Work out the finished part from the listing and answer in its coordinate system (mm). Coordinates: 2 decimals unless noted, no trailing zeros. Write each loop counter-clockwise with the first axis right and the second up, starting at its lowest first coordinate (ties: lowest second). Pieces come first, ordered by that corner, then holes. Notation, with made-up numbers: (88, 62.5) - (146, 62.5) arc R36 cw to (146, 100.5) - close; hole circle Ø7 at (-1.5, -17). An arc over 180 degrees is marked (long way). Use a Markdown table: item, result. Add a question column.
(1) The part is cut by section C-C, the plane z = -9. Give the vertices of the cut face in (x, y).
(2) The part is cut by section A-A, the plane y = 0.3. Give the vertices of the cut face in (x, z).
(3) For a pull along Y with two mould halves and no side action, classify faces 1 (the face through (-1, 1.016, -27)), 2 (the face through (-23.657, 0.751, 27.237)), 3 (the face through (-1, 0, -12)) as released by +Y, released by -Y, zero draft, split by the parting line, or undercut.
(4) Find the intervals of material crossed by line 1 (Y direction, x = -48, z = -41); line 2 (Z direction, x = 60, y = 0.5); line 3 (Z direction, x = -17, y = 0.2), in increasing order. Write a range as from..to.
(5) The part is cut by section D-D, the plane x = 32. Give the vertices of the cut face in (y, z).
(6) The part is cut by section B-B, the plane x = -10. Give the vertices of the cut face in (y, z), then the cut area to 3 significant figures.
(7) Given pin 1 Ø0.5 at (x, y) = (51, 0.5) entering from +Z; pin 2 Ø16.5 at (x, z) = (-21, -35.5) entering from +Y, each flat-ended and moving along its own axis, determine where each tip first touches the part or whether it passes through.
from build123d import *

# Parameters (mm, degrees)
F34_W     = 153.4406170249
F34_H     = 55.5722899735
F35_DEPTH = 0.762
F37_DEPTH = 1.27
F39_DEPTH = 0.254
F40_DEPTH = 0.254


# Not quite as in the source:
# - the program builds the solid bodies; features that only make, move or delete a surface that nothing else refers to are left out


with BuildPart() as f35:
    # F34 (on Front) → F35 (new body)
    with BuildSketch(Plane.XZ):
        with Locations((0.281136483, -27.7861449867)):
            Rectangle(F34_W, F34_H)
    extrude(amount=-F35_DEPTH)

    # F36 (on Front) → F37 (join)
    with BuildSketch(Plane.XZ):
        Polygon((41.6817590594, 0), (0, 55.2465841174), (-46.6600246727, 0), align=None)
    extrude(amount=-F37_DEPTH)

    # F38 (on face) → F39 (join)
    with BuildSketch(Plane(origin=(0, 1.27, 0), x_dir=(-1, 0, 0), z_dir=(0, 1, 0))):
        Polygon((46.6600246727, 0), (0, 55.2465841174), (-41.6817590594, 0), align=None)
    extrude(amount=F39_DEPTH)

    # F40 (add): a face of the model
    f40_faces = [f35.faces().sort_by_distance(p)[0] for p in [
        (0.281136483, 0.762, -27.7861449867),
    ]]
    extrude(f40_faces, amount=F40_DEPTH)


solid = f35.part
Model answer:
| question | item | result |
|---|---|---|
| 1 | outline | (-76.44, 0) - (77, 0) - (77, 1.02) - (-76.44, 1.02) - close |
| 2 | outline | (-76.44, -55.57) - (77, -55.57) - (77, 0) - (41.68, 0) - (0, 55.25) - (-46.66, 0) - (-76.44, 0) - close |
| 3 | face 1 | released by +Y |
| 3 | face 2 | zero draft |
| 3 | face 3 | released by -Y |
| 4 | line 1 | 0..1.02 |
| 4 | line 2 | -55.57..0 |
| 4 | line 3 | -55.57..35.12 |
| 5 | outline | (0, -55.57) - (1.02, -55.57) - (1.02, 0) - (1.52, 0) - (1.52, 12.83) - (0, 12.83) - close |
| 6 | outline | (0, -55.57) - (1.02, -55.57) - (1.02, 0) - (1.52, 0) - (1.52, 43.41) - (0, 43.41) - close |
| 6 | area | 123 mm^2 |
| 7 | pin 1 | z = 0 |
| 7 | pin 2 | y = 1.02 |
